Part print with two shaded views. Sizes in mm from the minimum x, y, z corner. A direction names the side the tool comes from. Give positions to 0.01 mm unless a question says otherwise; leave off trailing zeros. Write item = value, one per line. Start each with the question number.
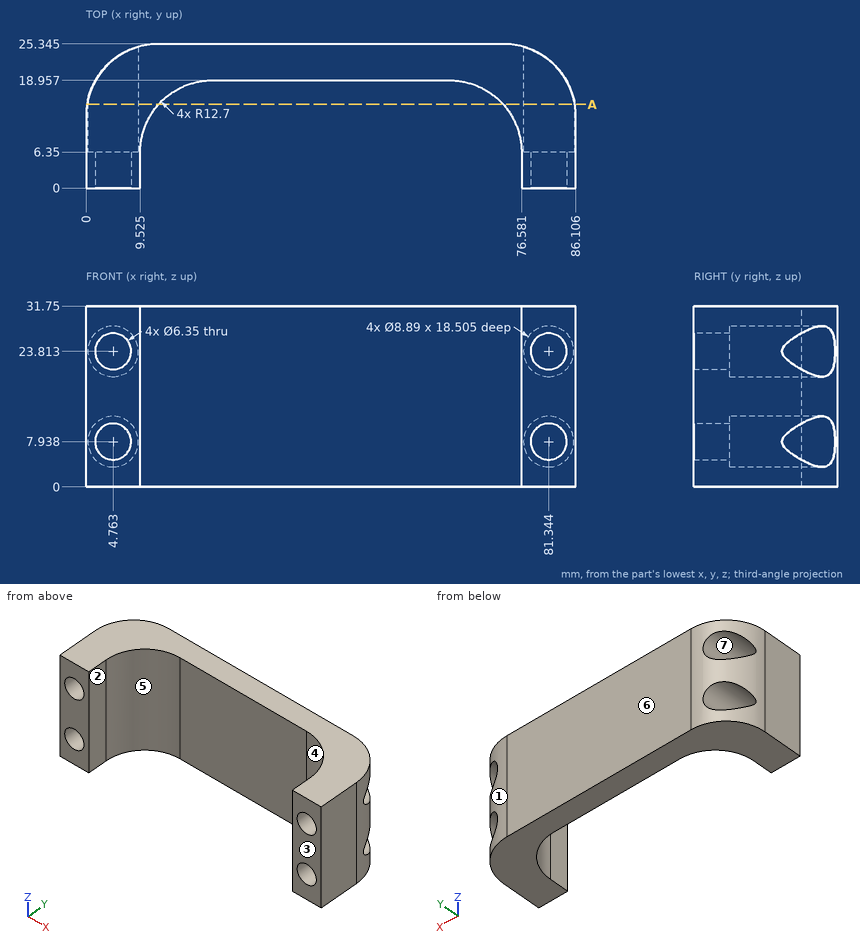
(1) 3-axis set-ups, long thin cutter, end or side, ignore diameter. For the marked faces 5, 6 and 7: which of +Z, -Z, +X, -X, +Y, -Y reach the whole face in a straight line?
(2) Flat gauge pins, fed straight in: P1, Ø4.5, axis at x = 4.5, z = 24, coming from the +Y side; P2, Ø14, axis at x = 81.34, z = 7.94, coming from the -Y side; P3, Ø9.5, axis at x = 48, z = 22, coming from the -Y side. Where does each tip first touch, or does it go through?
(3) Wall check: line 1 (X direction, y = 3, z = 9.5) (1 decimal); line 2 (X direction, y = 3, z = 14.5) (1 decimal); line 3 (Z direction, x = 79.5, y = 13.5). Give the ranges that are in metal, low to high. Write a range as [from, to].
(4) Mould opens along X. For the marked faces 1, 2, 3 and 4 say: released by +X, released by -X, zero draft, split by the parting line, or undercut.
(5) Cut at A-A, the plane y = 14.75. Give the number of separate pieces and of enclosed holes in the cut face.
Results:
q1.face_5 = +Z, -Z, -Y
q1.face_6 = +Z, -Z, +X, -X, +Y
q1.face_7 = +Y
q2.P1 = through
q2.P2 = 0
q2.P3 = 18.96
q3.line_1 = [0, 2], [7.5, 9.5], [76.6, 78.6], [84.1, 86.1]
q3.line_2 = [0, 9.5], [76.6, 86.1]
q3.line_3 = [0, 3.89], [11.98, 19.77], [27.86, 31.75]
q4.face_1 = released by +X
q4.face_2 = undercut
q4.face_3 = zero draft
q4.face_4 = undercut
q5.separate_pieces = 2
q5.enclosed_holes = 4
